Here's the drawing with two shaded views (mm, measured from the low corner). I have some questions. A direction names the side the tool comes from. Coordinates: 2 decimals unless noted, no trailing zeros. Write each loop counter-clockwise with the first axis right and the second up, starting at its lowest first coordinate (ties: lowest second). Pieces come first, ordered by that corner, then holes.
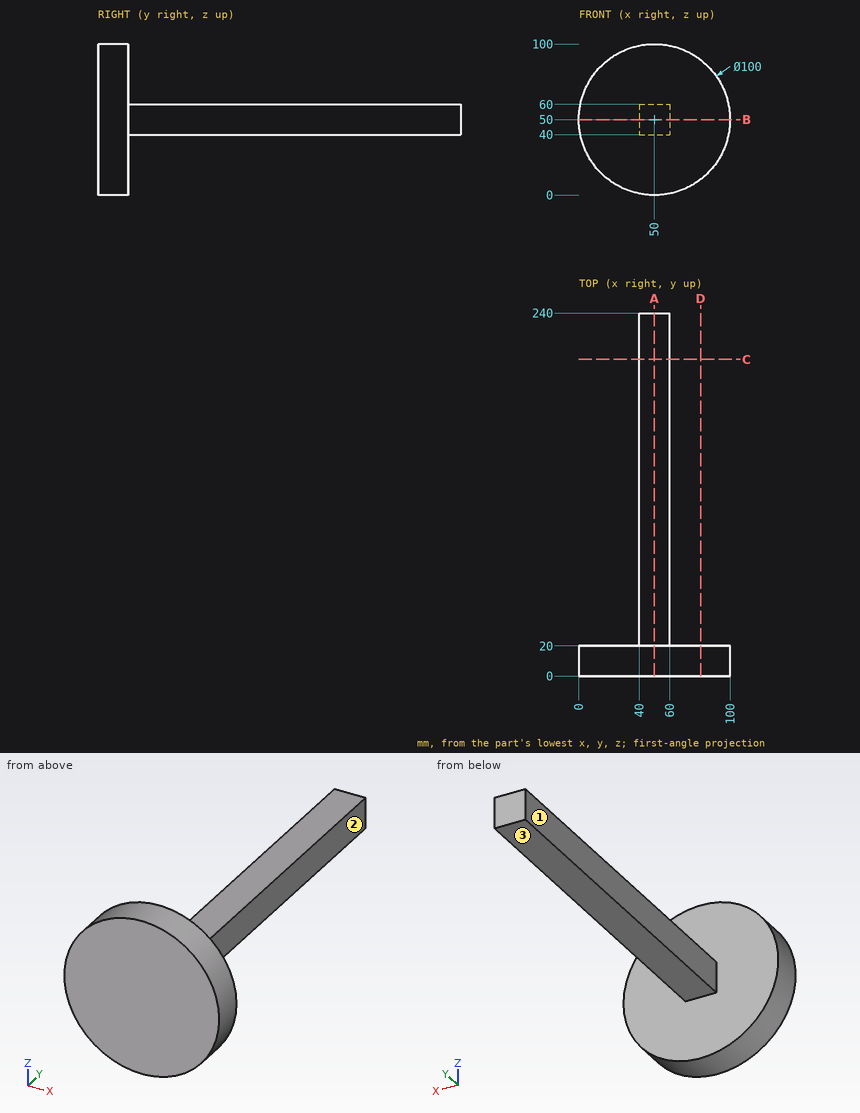
Item 1: If I drill on line 1 along Y through (x, z) = (42.5, 65); line 2 along X through (y, z) = (210.5, 56), over which ranges is the centre line in solid material (lowest first)?
Item 2: I want a section at B-B, the plane z = 50. List the corners of the cut face in (x, y) for me, then the cut area to 3 significant figures.
Item 3: Will these pins go through, and if not, where does the flat tip stop? pin 1 Ø1 at (x, z) = (55.5, 24.5) entering from +Y; pin 2 Ø22 at (x, y) = (48.5, 129.5) entering from -Z; pin 3 Ø16 at (y, z) = (147.5, 50) entering from +X; pin 4 Ø12 at (x, z) = (67, 61.5) entering from -Y.
Item 4: I want a section at A-A, the plane x = 50. List the corners of the cut face in (y, z) for me, then the cut area to 3 significant figures.
Item 5: I want a section at C-C, the plane y = 209.5. List the corners of the cut face in (x, z) for me.
Item 6: Which directions (+Z, -Z, +X, -X, +Y, -Y) give clear straight access to the entire face, cutting with the end or side of a thin tool? Please do the marked faces 1, 2 and 3.
Item 7: I want a section at D-D, the plane x = 80.5. List the corners of the cut face in (y, z) for me.
Taken from the geometry:
1. line 1: y = 0 to 20
1. line 2: x = 40 to 60
2. outline: (0, 0) - (100, 0) - (100, 20) - (60, 20) - (60, 240) - (40, 240) - (40, 20) - (0, 20) - close
2. area: 6,400 mm2
3. pin 1: stops at y = 20
3. pin 2: stops at z = 40
3. pin 3: stops at x = 60
3. pin 4: stops at y = 0
4. outline: (0, 0) - (20, 0) - (20, 40) - (240, 40) - (240, 60) - (20, 60) - (20, 100) - (0, 100) - close
4. area: 6,400 mm2
5. outline: (40, 40) - (60, 40) - (60, 60) - (40, 60) - close
6. face 1: +Z, -Z, -X, +Y
6. face 2: +Z, -Z, +X, +Y
6. face 3: -Z, +X, -X, +Y
7. outline: (0, 10.38) - (20, 10.38) - (20, 89.62) - (0, 89.62) - close
